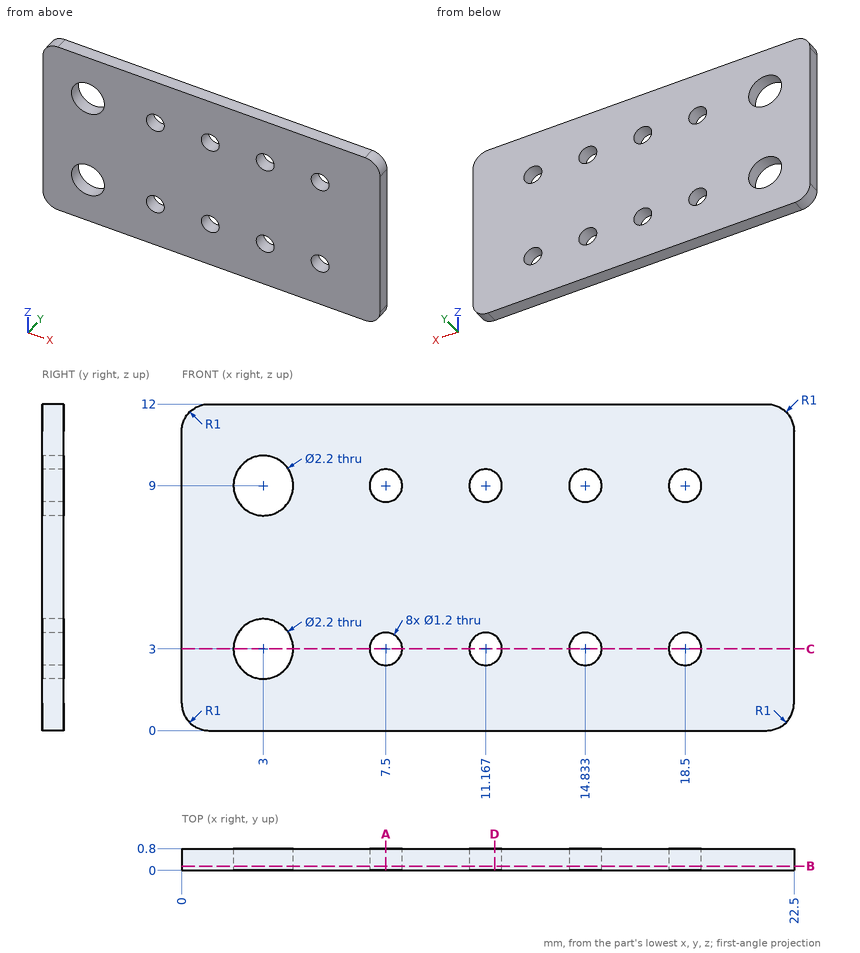
Study the drawing (mm; zero at the part's minimum x, y, z) and answer. Coordinates: 2 decimals unless noted, no trailing zeros. Write each loop counter-clockwise with the first axis right and the second up, starting at its lowest first coordinate (ties: lowest second). Pieces come first, ordered by that corner, then holes. Notation, with made-up numbers: (38, 16) - (58, 16) arc R29 ccw to (58, 50) - close; hole circle Ø9 at (-22.5, -16.75). An arc over 180 degrees is marked (long way). Answer as a JSON object with one key per item and string values. Group by question number.
1. A cutting plane is placed at A-A (x = 7.5). Determine the outline of the cut face in (y, z).
2. Consider L1, parallel to X at y = 0.6, z = 3.5 (1 decimal); L2, parallel to Z at x = 11.5, y = 0.05; L3, parallel to Z at x = 2.75, y = 0.55. Determine where each line is inside the solid, lowest interval first. Write a range as [from, to].
3. A cutting plane is placed at C-C (z = 3). Determine the outline of the cut face in (x, y), plus the area to 3 significant figures.
4. A cutting plane is placed at B-B (y = 0.15). Give the number of separate pieces and of enclosed holes in the cut face.
5. This flat-tipped pin is pushed along its axis until it touches: P1, Ø1.1, axis at x = 7.5, z = 9, coming from the -Y side (1 decimal). Where does it stop, or does it pass through?
6. A cutting plane is placed at D-D (x = 11.5). Determine the outline of the cut face in (y, z).
Worked out:
{
 "1": {"outline": "(0, 0) - (0.8, 0) - (0.8, 2.4) - (0, 2.4) - close; (0, 3.6) - (0.8, 3.6) - (0.8, 8.4) - (0, 8.4) - close; (0, 9.6) - (0.8, 9.6) - (0.8, 12) - (0, 12) - close"},
 "2": {"L1": "x = [0, 2], [4, 7.2], [7.8, 10.8], [11.5, 14.5], [15.2, 18.2], [18.8, 22.5]", "L2": "z = [0, 2.5], [3.5, 8.5], [9.5, 12]", "L3": "z = [0, 1.93], [4.07, 7.93], [10.07, 12]"},
 "3": {"outline": "(0, 0) - (1.9, 0) - (1.9, 0.8) - (0, 0.8) - close; (4.1, 0) - (6.9, 0) - (6.9, 0.8) - (4.1, 0.8) - close; (8.1, 0) - (10.57, 0) - (10.57, 0.8) - (8.1, 0.8) - close; (11.77, 0) - (14.23, 0) - (14.23, 0.8) - (11.77, 0.8) - close; (15.43, 0) - (17.9, 0) - (17.9, 0.8) - (15.43, 0.8) - close; (19.1, 0) - (22.5, 0) - (22.5, 0.8) - (19.1, 0.8) - close", "area": "12.4 mm²"},
 "4": {"separate pieces": "1", "enclosed holes": "10"},
 "5": {"P1": "passes through"},
 "6": {"outline": "(0, 0) - (0.8, 0) - (0.8, 2.5) - (0, 2.5) - close; (0, 3.5) - (0.8, 3.5) - (0.8, 8.5) - (0, 8.5) - close; (0, 9.5) - (0.8, 9.5) - (0.8, 12) - (0, 12) - close"}
}
